Source: CAD feature listing. Evaluate the final solid. Frame: model axes, mm. A direction names the side the tool comes from. Round coordinates to 2 decimals unless told otherwise and drop trailing zeros. Loops run counter-clockwise (first coordinate to the right, second up) from the corner with the lowest first, then second, coordinate; pieces in that order, holes last. Notation, with made-up numbers: M 29,61.25 L 68,61.25 A16 cw 68,85.25 Z; hole C 49,44 d9. An arc over 180 degrees is marked long. Write each question's results on one line, items separated by ' | '. Start each with the question number.
1. Ray query, line 1 (Y direction, x = 0, z = -6.75); line 2 (X direction, y = 79, z = 2.25); line 3 (X direction, y = 139.5, z = -6.9). Return the intervals inside material, ascending.
2. Set-up query: faces 4 (the flat face through (0, 99, 6.5)), 5 (the flat face through (0, 99, -7.5)). Return all of +Z, -Z, +X, -X, +Y, -Y with unobstructed straight access to the full face (end or side cutting, diameter ignored); none if empty.
3. Draft query along X for faces 1 (the flat face through (-0.1, 7.6, 6.8)), 2 (the flat face through (-6.5, 106, 0)), 3 (the flat face through (-7, 200, 0)). Return one class per face: released by +X, released by -X, zero draft, split by the parting line, or undercut.
4. Section A-A on y = 70.5. Output: boundary loops of the cut face in (x, z).
5. Section B-B on z = 4.25. Output: boundary loops of the cut face in (x, y), and give its area (3 significant figures).
6. Contact query for flat-ended pins moving along their axis: pin 1 Ø1.8 at (x, y) = (0, 139.5) entering from +Z; pin 2 Ø5 at (y, z) = (177.5, 0) entering from -X. Output: stop coordinate, or through.
from build123d import *

# Parameters (mm, degrees)
SKETCH_1_W          = 15
SKETCH_1_H          = 15
SKETCH_1_W_2        = 13
SKETCH_1_H_2        = 13
EXTRUDE_1_DEPTH     = 200
SKETCH_2_R          = 1.5
CUT_EXTRUDE_1_DEPTH = 201.701893364
SKETCH_3_R          = 1.5
CUT_EXTRUDE_2_DEPTH = 201.701893364


with BuildPart() as part:
    # 草图1 → 凸台-拉伸1 (new body)
    with BuildSketch(Plane(origin=(0, 0, 0), x_dir=(1, 0, 0), z_dir=(0, 1, 0))):
        Rectangle(SKETCH_1_W, SKETCH_1_H)
        Rectangle(SKETCH_1_W_2, SKETCH_1_H_2, mode=Mode.SUBTRACT)
    extrude(amount=EXTRUDE_1_DEPTH)

    # 草图2 → 切除-拉伸1 (cut, through all)
    with BuildSketch(Plane.XY.offset(7.5)):
        with Locations((0, 37.5)):
            Circle(SKETCH_2_R)
        with Locations((0, 17.5)):
            Circle(SKETCH_2_R)
        with Locations((0, 57.5)):
            Circle(SKETCH_2_R)
        with Locations((0, 187.5)):
            Circle(SKETCH_2_R)
        with Locations((0, 139.5)):
            Circle(SKETCH_2_R)
        Polygon((7.5, 0), (-7.5, 0), (-7.5, 15), align=None)
    extrude(amount=-CUT_EXTRUDE_1_DEPTH, mode=Mode.SUBTRACT)

    # 草图3 → 切除-拉伸2 (cut, through all)
    with BuildSketch(Plane(origin=(7.5, 0, 0), x_dir=(0, 0, -1), z_dir=(1, 0, 0))):
        with Locations((0, 157.5)):
            Circle(SKETCH_3_R)
        with Locations((0, 177.5)):
            Circle(SKETCH_3_R)
        with Locations((0, 132.5)):
            Circle(SKETCH_3_R)
        with Locations((0, 187.5)):
            Circle(SKETCH_3_R)
    extrude(amount=-CUT_EXTRUDE_2_DEPTH, mode=Mode.SUBTRACT)


solid = part.part
Taken from the geometry:
1) line 1: 7.5 to 16, 19 to 36, 39 to 56, 59 to 138, 141 to 186, 189 to 200 | line 2: -7.5 to -6.5, 6.5 to 7.5 | line 3: -7.5 to -1.5, 1.5 to 7.5
2) face 4: +Y, -Y | face 5: -Z, +X, -X, +Y, -Y
3) face 1: released by -X | face 2: undercut | face 3: zero draft
4) outline: M -7.5,-7.5 L 7.5,-7.5 L 7.5,7.5 L -7.5,7.5 Z; hole M -6.5,-6.5 L 6.5,-6.5 L 6.5,6.5 L -6.5,6.5 Z
5) outline: M -7.5,15 L -6.5,14 L -6.5,200 L -7.5,200 Z; M 6.5,1 L 7.5,0 L 7.5,200 L 6.5,200 Z | area: 385 mm^2
6) pin 1: through | pin 2: x = -7.5
